from build123d import *

# Parameters (mm, degrees)
F1_DEPTH = 203.2
F2_DEPTH = 406.4


with BuildPart() as f1:
    # F0 (on Front) → F1 (new body)
    with BuildSketch(Plane.XZ):
        with BuildLine():
            Line((-670.171326, 139.884379), (-670.171326, 114.484379))
            ThreePointArc((-670.171326, 114.484379), (-580.368765, 77.28694), (-543.171326, -12.515621))
            ThreePointArc((-543.171326, -12.515621), (-580.368765, -102.318182), (-670.171326, -139.515621))
            Line((-670.171326, -139.515621), (-670.171326, -164.915621))
            Line((-670.171326, -164.915621), (684.760069, -164.915621))
            Line((684.760069, -164.915621), (684.760069, -139.515621))
            ThreePointArc((684.760069, -139.515621), (557.760069, -12.515621), (684.760069, 114.484379))
            Line((684.760069, 114.484379), (684.760069, 139.884379))
            Line((684.760069, 139.884379), (-670.171326, 139.884379))
        make_face()
        with BuildLine():
            ThreePointArc((-670.171326, -139.515621), (-797.171326, -12.515621), (-670.171326, 114.484379))
            Line((-670.171326, 114.484379), (-670.171326, 139.884379))
            ThreePointArc((-670.171326, 139.884379), (-822.571326, -12.515621), (-670.171326, -164.915621))
            Line((-670.171326, -164.915621), (-670.171326, -139.515621))
        make_face()
        with BuildLine():
            ThreePointArc((684.760069, -164.915621), (837.160069, -12.515621), (684.760069, 139.884379))
            Line((684.760069, 139.884379), (684.760069, 114.484379))
            ThreePointArc((684.760069, 114.484379), (774.562631, 77.28694), (811.760069, -12.515621))
            ThreePointArc((811.760069, -12.515621), (774.562631, -102.318182), (684.760069, -139.515621))
            Line((684.760069, -139.515621), (684.760069, -164.915621))
        make_face()
    extrude(amount=F1_DEPTH)

    # F0 (on Front) → F2 (join)
    with BuildSketch(Plane.XZ):
        with BuildLine():
            ThreePointArc((811.760069, -12.515621), (774.562631, 77.28694), (684.760069, 114.484379))
            Line((684.760069, 114.484379), (684.760069, -139.515621))
            ThreePointArc((684.760069, -139.515621), (774.562631, -102.318182), (811.760069, -12.515621))
        make_face()
        with BuildLine():
            Line((684.760069, -139.515621), (684.760069, 114.484379))
            ThreePointArc((684.760069, 114.484379), (557.760069, -12.515621), (684.760069, -139.515621))
        make_face()
    extrude(amount=F2_DEPTH)


solid = f1.part
Design review of the part built by this model. Coordinates are the model's own, in mm. Give positions to 0.01 mm unless a question says otherwise; leave off trailing zeros. Order: outer loops, then holes, each group sorted by start corner. A loop starts at its lowest first (then second) coordinate and runs counter-clockwise, first axis right, second up.
1. For pin 1 Ø1.5 at (y, z) = (-155.5, -8) entering from -X; pin 2 Ø1 at (y, z) = (-49, -59.5) entering from -X; pin 3 Ø5 at (y, z) = (-216.5, 32) entering from +X, all flat-tipped, find the tip position at first contact; note any pin that passes through.
Solution:
pin 1: stops at x = -822.52
pin 2: stops at x = -815.31
pin 3: stops at x = 804.61
2. To check wall thickness, follow L1, parallel to Y at x = 11, z = -85.5; L2, parallel to X at y = -132.5, z = -45; L3, parallel to X at y = -43, z = -44.5. State the ranges of each line that lie inside material, in increasing order.
Solution:
L1: y = -203.2 to 0
L2: x = -819.07 to -792.95, -547.4 to 833.66
L3: x = -819.18 to -793.08, -547.26 to 833.77
3. Add section C-C, the plane x = 590. State the section outline as (y, z) points.
Solution:
outline: (-406.4, -97.07) - (-203.2, -97.07) - (-203.2, -164.92) - (0, -164.92) - (0, 139.88) - (-203.2, 139.88) - (-203.2, 72.04) - (-406.4, 72.04) - close
4. Add section B-B, the plane z = -62.5. State the section outline as (x, y) points, then the cut area to 3 significant figures.
Solution:
outline: (-814.14, -203.2) - (-786.92, -203.2) - (-786.92, 0) - (-814.14, 0) - close; (-553.42, -203.2) - (568.01, -203.2) - (568.01, -406.4) - (801.51, -406.4) - (801.51, -203.2) - (828.73, -203.2) - (828.73, 0) - (-553.42, 0) - close
area: 334,000 mm2
5. Add section A-A, the plane y = -174. State the section outline as (x, z) points, then the cut area to 3 significant figures.
Solution:
outline: (-670.17, -164.92) - (684.76, -164.92) arc R152.4 ccw to (684.76, 139.88) - (-670.17, 139.88) arc R152.4 ccw to start; hole (-670.17, -139.52) arc R127 ccw to (-543.17, -12.52) arc R127 ccw (long way) to start
area: 435,000 mm2
6. Add section D-D, the plane z = 87. State the section outline as (x, y) points, then the cut area to 3 significant figures.
Solution:
outline: (-785.59, -203.2) - (-749.07, -203.2) - (-749.07, 0) - (-785.59, 0) - close; (-591.27, -203.2) - (605.86, -203.2) - (605.86, -406.4) - (763.66, -406.4) - (763.66, -203.2) - (800.18, -203.2) - (800.18, 0) - (-591.27, 0) - close
area: 322,000 mm2
